```python
from build123d import *

# Parameters (mm, degrees)
SKETCH1_R               = 19.05
BOSS_EXTRUDE1_DEPTH     = 12.7
CUT_EXTRUDE1_DEPTH      = 6.35
CUT_EXTRUDE3_DEPTH      = 126.437752774
CUT_EXTRUDE3_DEPTH_BACK = 126.437752774
SKETCH4_R               = 2.159


with BuildPart() as part:
    # Sketch1 → Boss-Extrude1 (new body)
    with BuildSketch(Plane(origin=(0, 0, 0), x_dir=(0, 0, -1), z_dir=(1, 0, 0))):
        with BuildLine():
            Line((25.4, 62.611), (-25.4, 62.611))
            ThreePointArc((-25.4, 62.611), (-43.71389723, 59.350669702), (-59.777434529, 49.970298982))
            Line((-59.777434529, 49.970298982), (-101.281034529, 14.478))
            ThreePointArc((-101.281034529, 14.478), (-80.929937509, 17.302618411), (-69.85, 0))
            ThreePointArc((-69.85, 0), (-80.929937509, -17.302618411), (-101.281034529, -14.478))
            Line((-101.281034529, -14.478), (-59.777434529, -49.970298982))
            ThreePointArc((-59.777434529, -49.970298982), (-43.71389723, -59.350669702), (-25.4, -62.611))
            Line((-25.4, -62.611), (25.4, -62.611))
            ThreePointArc((25.4, -62.611), (43.699078076, -59.34404997), (59.737214243, -49.946847768))
            Line((59.737214243, -49.946847768), (101.269374674, -14.487973703))
            ThreePointArc((101.269374674, -14.487973703), (69.85, -7.706e-06), (101.269379322, 14.48794821))
            Line((101.269379322, 14.48794821), (59.737230268, 49.9468356))
            ThreePointArc((59.737230268, 49.9468356), (43.699087699, 59.344046737), (25.4, 62.611))
        make_face()
        with Locations((88.9, -1.0762e-05)):
            Circle(SKETCH1_R)
        with Locations((-88.9, 0)):
            Circle(SKETCH1_R)
    extrude(amount=BOSS_EXTRUDE1_DEPTH)

    # Sketch2 → Cut-Extrude1 (cut)
    with BuildSketch(Plane(origin=(12.7, 0, 0), x_dir=(0, 0, -1), z_dir=(1, 0, 0))):
        with BuildLine():
            Line((-49.889980522, 38.373041727), (-93.122597105, 5.564161993))
            ThreePointArc((-93.122597105, 5.564161993), (-95.885, 0), (-93.122597105, -5.564161993))
            Line((-93.122597105, -5.564161993), (-49.889980522, -38.373041727))
            ThreePointArc((-49.889980522, -38.373041727), (-38.445328657, -45.050322999), (-25.4, -47.371))
            Line((-25.4, -47.371), (25.4, -47.371))
            ThreePointArc((25.4, -47.371), (38.425542458, -45.045538785), (49.841714504, -38.356477415))
            Line((49.841714504, -38.356477415), (93.118252802, -5.56746694))
            ThreePointArc((93.118252802, -5.56746694), (95.885, -1.1883e-05), (93.118254588, 5.567444063))
            Line((93.118254588, 5.567444063), (49.84172681, 38.356468422))
            ThreePointArc((49.84172681, 38.356468422), (38.425549787, 45.045536399), (25.4, 47.371))
            Line((25.4, 47.371), (-25.4, 47.371))
            ThreePointArc((-25.4, 47.371), (-38.445328657, 45.050322999), (-49.889980522, 38.373041727))
        make_face()
    extrude(amount=-CUT_EXTRUDE1_DEPTH, mode=Mode.SUBTRACT)

    # Sketch4 → Cut-Extrude3 (cut, two sides: drawn at the far end of the back side and taken through both)
    with BuildSketch(Plane(origin=(12.7, 0, 0), x_dir=(0, 0, -1), z_dir=(1, 0, 0)).offset(-CUT_EXTRUDE3_DEPTH_BACK)):
        with BuildLine():
            ThreePointArc((-73.940141084, 27.832575617), (-76.984164998, 28.070231704), (-77.221821084, 25.02620779))
            Line((-77.221821084, 25.02620779), (-73.940141084, 27.832575617))
        make_face()
        with BuildLine():
            Line((-73.940141084, 27.832575617), (-77.221821084, 25.02620779))
            ThreePointArc((-77.221821084, 25.02620779), (-74.833081546, 24.404070178), (-73.421981084, 26.429391704))
            ThreePointArc((-73.421981084, 26.429391704), (-73.555659559, 27.177291242), (-73.940141084, 27.832575617))
        make_face()
        with Locations((-54.833341451, 44.171983407)):
            Circle(SKETCH4_R)
        with Locations((-30.48, 54.706186836)):
            Circle(SKETCH4_R)
        with Locations((0, 54.991)):
            Circle(SKETCH4_R)
        with Locations((30.478659799, 54.70517335)):
            Circle(SKETCH4_R)
        with Locations((54.789478539, 44.151652011)):
            Circle(SKETCH4_R)
        with Locations((75.555553066, 26.422208316)):
            Circle(SKETCH4_R)
        with Locations((92.827553066, 14.992208316)):
            Circle(SKETCH4_R)
        with Locations((92.827553066, -14.992208316)):
            Circle(SKETCH4_R)
        with Locations((75.555553066, -26.422208316)):
            Circle(SKETCH4_R)
        with Locations((54.789478539, -44.151652011)):
            Circle(SKETCH4_R)
        with Locations((30.478659799, -54.70517335)):
            Circle(SKETCH4_R)
        with Locations((0, -54.991)):
            Circle(SKETCH4_R)
        with Locations((-30.48, -54.706186836)):
            Circle(SKETCH4_R)
        with Locations((-54.833341451, -44.171983407)):
            Circle(SKETCH4_R)
        with Locations((-75.580981084, -26.429391704)):
            Circle(SKETCH4_R)
        with Locations((-92.852981084, -14.999391704)):
            Circle(SKETCH4_R)
        with Locations((-92.852981084, 14.999391704)):
            Circle(SKETCH4_R)
    extrude(amount=CUT_EXTRUDE3_DEPTH + CUT_EXTRUDE3_DEPTH_BACK, mode=Mode.SUBTRACT)


solid = part.part
```
Could you check a few things on this model? Use its own coordinates, in mm. A direction names the side the tool comes from. Coordinates: 2 decimals unless noted, no trailing zeros. Write each loop counter-clockwise with the first axis right and the second up, starting at its lowest first coordinate (ties: lowest second). Pieces come first, ordered by that corner, then holes. Notation, with made-up numbers: (34, 80.5) - (64, 80.5) arc R24 ccw to (64, 114.5) - close; hole circle Ø7 at (-33.5, 40). An arc over 180 degrees is marked (long way). Use a Markdown table: item, result.
Q1. Imagine slicing it at B-B (y = -35.5). List the corners of the cut face in (x, z) for me.
Geometry check:
| item | result |
|---|---|
| outline | (0, -76.66) - (12.7, -76.66) - (12.7, -53.61) - (6.35, -53.61) - (6.35, 53.68) - (12.7, 53.68) - (12.7, 76.7) - (0, 76.7) - close |
Q2. Which directions (+Z, -Z, +X, -X, +Y, -Y) give clear straight access to the entire face, cutting with the end or side of a thin tool? Please do faces 1 (the cylindrical face through (9.57, -45.11, -38.25)), 2 (the cylindrical face through (6.261, -14.351, 90.794)).
Geometry check:
| item | result |
|---|---|
| face 1 | +X |
| face 2 | +X, -X |
Q3. Thinking about a two-plate mould opening in Z: for faces 3 (the cylindrical face through (6.26, -57.1, 0.47)), 4 (the flat face through (6.26, -32.47, -80.21)), 5 (the flat face through (12.7, -51, 9)), which applies, +Z half, -Z half, draft (parallel to the pull), parting line (faces both ways), or undercut?
Geometry check:
| item | result |
|---|---|
| face 3 | undercut |
| face 4 | -Z half |
| face 5 | draft |
Q4. Please list where these lines run through material, in increasing order: L1, parallel to Y at x = 6, z = -1; L2, parallel to Z at x = 4, y = 28; L3, parallel to Z at x = 1.25, y = -14.
Geometry check:
| item | result |
|---|---|
| L1 | y = -62.61 to -56.9, -53.08 to 53.08, 56.9 to 62.61 |
| L2 | z = -85.44 to -77.03, -74.08 to 74.1, 77.06 to 85.47 |
| L3 | z = -101.82 to -94.75, -90.91 to 90.94, 94.77 to 101.82 |
Q5. Imagine slicing it at C-C (z = 30.48). List the corners of the cut face in (x, y) for me, and give its area (3 significant figures).
Geometry check:
| item | result |
|---|---|
| outline | (0, -62.37) - (12.7, -62.37) - (12.7, -56.87) - (0, -56.87) - close; (0, -52.55) - (12.7, -52.55) - (12.7, -47.03) - (6.35, -47.03) - (6.35, 47.03) - (12.7, 47.03) - (12.7, 52.55) - (0, 52.55) - close; (0, 56.87) - (12.7, 56.87) - (12.7, 62.37) - (0, 62.37) - close |
| area | 877 mm2 |
Q6. Imagine slicing it at A-A (z = 0). List the corners of the cut face in (x, y) for me, and give its area (3 significant figures).
Geometry check:
| item | result |
|---|---|
| outline | (0, -62.61) - (12.7, -62.61) - (12.7, -57.15) - (0, -57.15) - close; (0, -52.83) - (12.7, -52.83) - (12.7, -47.37) - (6.35, -47.37) - (6.35, 47.37) - (12.7, 47.37) - (12.7, 52.83) - (0, 52.83) - close; (0, 57.15) - (12.7, 57.15) - (12.7, 62.61) - (0, 62.61) - close |
| area | 879 mm2 |
Q7. I'm going to push flat-ended pins straight in: pin 1 Ø8 at (y, z) = (-25.5, 2) entering from +X; pin 2 Ø1 at (x, y) = (5, -27.5) entering from +Z; pin 3 Ø1 at (x, y) = (4, -42.5) entering from +Z. Where does each tip first touch, or does it pass through?
Geometry check:
| item | result |
|---|---|
| pin 1 | stops at x = 6.35 |
| pin 2 | stops at z = 86.64 |
| pin 3 | stops at z = 69.1 |
Q8. Imagine slicing it at D-D (x = 9.75). Count the separate pieces of the cut face and the enclosed holes in it, and give its area (3 significant figures).
Geometry check:
| item | result |
|---|---|
| separate pieces | 1 |
| enclosed holes | 19 |
| area | 6,760 mm2 |
